```python
from build123d import *

# Parameters (mm, degrees)
EXTRUDE_1_DEPTH = 8.5
SKETCH_1_6_R    = 2.75
EXTRUDE_2_DEPTH = 8
EXTRUDE_START   = -2
EXTRUDE_3_DEPTH = 2
FILLET_4_R      = 0.3
FILLET_1_R      = 2
CHAMFER_1_SIZE  = 0.2
FILLET_2_R      = 2
FILLET_3_SIZE   = 5
FILLET_3_SIZE_2 = 5.5
EXTRUDE_START_2 = 4
EXTRUDE_4_DEPTH = 4


with BuildPart() as part:
    # Sketch 1 → Extrude 1 (new body)
    with BuildSketch(Plane.XY):
        with BuildLine():
            ThreePointArc((-15, 13), (-14.414213562, 14.414213562), (-13, 15))
            Line((-13, 15), (13, 15))
            ThreePointArc((13, 15), (14.414213562, 14.414213562), (15, 13))
            Line((15, 13), (15, -13))
            ThreePointArc((15, -13), (14.414213562, -14.414213562), (13, -15))
            Line((13, -15), (-13, -15))
            ThreePointArc((-13, -15), (-14.414213562, -14.414213562), (-15, -13))
            Line((-15, -13), (-15, 13))
        make_face()
        with BuildLine():
            ThreePointArc((-13, -11), (-12.414213562, -12.414213562), (-11, -13))
            Line((-11, -13), (11, -13))
            ThreePointArc((11, -13), (12.414213562, -12.414213562), (13, -11))
            Line((13, -11), (13, 11))
            ThreePointArc((13, 11), (12.414213562, 12.414213562), (11, 13))
            Line((11, 13), (-11, 13))
            ThreePointArc((-11, 13), (-12.414213562, 12.414213562), (-13, 11))
            Line((-13, 11), (-13, -11))
        make_face(mode=Mode.SUBTRACT)
    extrude(amount=EXTRUDE_1_DEPTH)



with BuildPart() as body_2:
    # Sketch 1_6 → Extrude 2 (new body)
    with BuildSketch(Plane.XY):
        Circle(SKETCH_1_6_R)
        Polygon((-2.085, -0.585), (-2.085, 0.585), (-0.585, 0.585), (-0.585, 2.085), (0.585, 2.085), (0.585, 0.585), (2.085, 0.585), (2.085, -0.585), (0.585, -0.585), (0.585, -2.085), (-0.585, -2.085), (-0.585, -0.585), align=None, mode=Mode.SUBTRACT)
    extrude(amount=EXTRUDE_2_DEPTH)


with BuildPart() as part_1:
    add(part.part)

    add(body_2.part)  # Extrude 3 merges body 2
    # Sketch 1_7 → Extrude 3 (add)
    with BuildSketch(Plane.XY.offset(EXTRUDE_START)):
        with BuildLine():
            Line((-13, 15), (13, 15))
            ThreePointArc((13, 15), (14.414213562, 14.414213562), (15, 13))
            Line((15, 13), (15, -13))
            ThreePointArc((15, -13), (14.414213562, -14.414213562), (13, -15))
            Line((13, -15), (-13, -15))
            ThreePointArc((-13, -15), (-14.414213562, -14.414213562), (-15, -13))
            Line((-15, -13), (-15, 13))
            ThreePointArc((-15, 13), (-14.414213562, 14.414213562), (-13, 15))
        make_face()
    extrude(amount=EXTRUDE_3_DEPTH)

    # Fillet 4
    fillet_4_edges = [part_1.edges().sort_by_distance(p)[0] for p in [
        (0.585, 0.585, 4),
        (0.585, -0.585, 4),
        (-0.585, -0.585, 4),
        (-0.585, 0.585, 4),
    ]]
    fillet(fillet_4_edges, radius=FILLET_4_R)

    # Fillet 1
    fillet_1_edges = [part_1.edges().sort_by_distance(p)[0] for p in [
        (-14.414213562, -14.414213562, -2),
        (-15, 0, -2),
        (14.414213562, 14.414213562, -2),
        (14.414213562, -14.414213562, -2),
        (0, -15, -2),
        (-14.414213562, 14.414213562, -2),
        (0, 15, -2),
        (15, 0, -2),
    ]]
    fillet(fillet_1_edges, radius=FILLET_1_R)

    # Chamfer 1
    chamfer_1_edges = [part_1.edges().sort_by_distance(p)[0] for p in [
        (1.485, 0.585, 8),
        (1.485, -0.585, 8),
        (0.585, -1.485, 8),
        (-0.585, -1.485, 8),
        (0.672867966, -0.672867966, 8),
        (-0.672867966, -0.672867966, 8),
        (0.672867966, 0.672867966, 8),
        (-0.672867966, 0.672867966, 8),
        (0, -2.085, 8),
        (-1.485, -0.585, 8),
        (-2.085, 0, 8),
        (-0.585, 1.485, 8),
        (0, 2.085, 8),
        (0.585, 1.485, 8),
        (2.085, 0, 8),
        (-1.485, 0.585, 8),
    ]]
    chamfer(chamfer_1_edges, length=CHAMFER_1_SIZE)

    # Fillet 2
    fillet_2_edges = [part_1.edges().sort_by_distance(p)[0] for p in [
        (0, -13, 0),
        (12.414213562, -12.414213562, 0),
        (13, 0, 0),
        (12.414213562, 12.414213562, 0),
        (0, 13, 0),
        (-12.414213562, 12.414213562, 0),
        (-13, 0, 0),
        (-12.414213562, -12.414213562, 0),
    ]]
    fillet(fillet_2_edges, radius=FILLET_2_R)

    # Fillet 3
    # a fillet whose section is not a circle: 5.5, 5 mm, written as the material it adds along each edge
    with BuildSketch(Plane(origin=(0, 0, 0), x_dir=(1, 0, 0), z_dir=(0, -1, 0))) as fillet_3_piece_1:
        with BuildLine():
            Bezier((2.75 + FILLET_3_SIZE, 0), (2.75, 0), (2.75, FILLET_3_SIZE_2), weights=[1, 0.333333333, 1])
            Line((2.75, FILLET_3_SIZE_2), (2.75, 0))
            Line((2.75, 0), (2.75 + FILLET_3_SIZE, 0))
        make_face()
    revolve(axis=Axis((0, 0, 0), (0, 0, 1)))

    # Sketch 3 → Extrude 4 (add)
    with BuildSketch(Plane.XY.offset(EXTRUDE_START_2)):
        with BuildLine():
            Line((0.585, 0.885), (0.585, 2.085))
            Line((0.585, 2.085), (-0.585, 2.085))
            Line((-0.585, 2.085), (-0.585, 0.885))
            ThreePointArc((-0.585, 0.885), (-0.672867966, 0.672867966), (-0.885, 0.585))
            Line((-0.885, 0.585), (-2.085, 0.585))
            Line((-2.085, 0.585), (-2.085, -0.585))
            Line((-2.085, -0.585), (-0.885, -0.585))
            ThreePointArc((-0.885, -0.585), (-0.672867966, -0.672867966), (-0.585, -0.885))
            Line((-0.585, -0.885), (-0.585, -2.085))
            Line((-0.585, -2.085), (0.585, -2.085))
            Line((0.585, -2.085), (0.585, -0.885))
            ThreePointArc((0.585, -0.885), (0.672867966, -0.672867966), (0.885, -0.585))
            Line((0.885, -0.585), (2.085, -0.585))
            Line((2.085, -0.585), (2.085, 0.585))
            Line((2.085, 0.585), (0.885, 0.585))
            ThreePointArc((0.885, 0.585), (0.672867966, 0.672867966), (0.585, 0.885))
        make_face()
    extrude(amount=-EXTRUDE_4_DEPTH)


solid = part_1.part
```
Here's how the part is built. I have some questions about the finished solid (model axes, mm). A direction names the side the tool comes from. Coordinates: 2 decimals unless noted, no trailing zeros. Loops run counter-clockwise (first coordinate to the right, second up) from the corner with the lowest first, then second, coordinate; pieces in that order, holes last. Notation, with made-up numbers: M -33,-39 L 0,-39 A24 ccw 0,-1 Z; hole C 20,40.5 d10. An arc over 180 degrees is marked long. One line per item, written item: value.
1. Please list where these lines run through material, in increasing order: probe 1 along Y at (x, z) = (4.5, 6.5); probe 2 along Y at (x, z) = (-3, 3.75).
Geometry says:
probe 1: y = -15 to -13, 13 to 15
probe 2: y = -15 to -13, -1.54 to 1.54, 13 to 15
2. Imagine slicing it at B-B (y = 10.5). List the corners of the cut face in (x, z) for me.
Geometry says:
outline: M -15,0 A2 ccw -13,-2 L 13,-2 A2 ccw 15,0 L 15,8.5 L 13,8.5 L 13,2 A2 cw 11,0 L -11,0 A2 cw -13,2 L -13,8.5 L -15,8.5 Z
3. On a 3-axis mill with a long thin cutter (end or side, diameter ignored), from which of +Z, -Z, +X, -X, +Y, -Y can I reach the whole of each face in a straight line? I mean faces 1 (the flat face through (14, 0, 8.5)), 2 (the flat face through (0, 0, 4)). Say none if no direction works.
Geometry says:
face 1: +Z, +X, -X, +Y, -Y
face 2: +Z
4. Thinking about a two-plate mould opening in Y: for faces 3 (the flat face through (15, 0, 4)), 4 (the flat face through (0, 15, 4)), 5 (the flat face through (0, -2.085, 6)), which applies, +Y half, -Y half, draft (parallel to the pull), parting line (faces both ways), or undercut?
Geometry says:
face 3: draft
face 4: +Y half
face 5: undercut
5. Will these pins go through, and if not, where does the flat tip stop? pin 1 Ø1.6 at (x, y) = (1.5, 0.5) entering from +Z; pin 2 Ø1.3 at (x, y) = (0, 1) entering from +Z (3 decimals); pin 3 Ø6 at (x, y) = (5.5, -6.5) entering from +Z.
Geometry says:
pin 1: stops at z = 8
pin 2: stops at z = 7.865
pin 3: stops at z = 1.19
6. Imagine slicing it at A-A (z = 6.25). State how many separate pieces and enclosed holes the cut face has, and give its area (3 significant figures).
Geometry says:
separate pieces: 2
enclosed holes: 2
area: 239 mm2
